from build123d import *

# Parameters (mm, degrees)
SKETCH1_R           = 3.048
BOSS_EXTRUDE1_DEPTH = 1.905
CUT_EXTRUDE1_DEPTH  = 1.651
BOSS_EXTRUDE2_START = 1.27
BOSS_EXTRUDE2_DEPTH = 1.27


with BuildPart() as part:
    # Sketch1 → Boss-Extrude1 (new body)
    with BuildSketch(Plane.XY):
        with BuildLine():
            Line((-5.49275, -17.49425), (-5.49275, -22.42185))
            Line((-5.49275, -22.42185), (-4.90855, -23.59025))
            Line((-4.90855, -23.59025), (-6.02615, -30.95625))
            ThreePointArc((-6.02615, -30.95625), (-5.598504604, -32.704973448), (-3.99415, -33.52165))
            ThreePointArc((-3.99415, -33.52165), (-0.284785682, -32.892281616), (3.42265, -32.25165))
            Line((3.42265, -32.25165), (4.94665, -24.09825))
            ThreePointArc((4.94665, -24.09825), (2.651841734, -25.057223226), (2.50825, -22.57425))
            ThreePointArc((2.50825, -22.57425), (2.10181036, -20.83747495), (2.73685, -19.17065))
            ThreePointArc((2.73685, -19.17065), (4.08470653, -17.176398636), (6.47065, -17.49425))
            ThreePointArc((6.47065, -17.49425), (7.46828342, -1.95088497), (5.45465, 13.49375))
            ThreePointArc((5.45465, 13.49375), (5.282315002, 20.474416107), (6.92785, 27.26055))
            ThreePointArc((6.92785, 27.26055), (5.106547792, 33.02758949), (-0.64135, 31.14675))
            Line((-0.64135, 31.14675), (-2.67335, 13.36675))
            Line((-2.67335, 13.36675), (-4.95935, 11.20775))
            Line((-4.95935, 11.20775), (-6.12775, -4.03225))
            Line((-6.12775, -4.03225), (-3.07975, -8.27405))
            Line((-3.07975, -8.27405), (-3.84175, -16.22425))
            Line((-3.84175, -16.22425), (-5.49275, -17.49425))
        make_face()
        with Locations(Location((3.16865, 29.24175, 0), (0, 0, 180))):
            Circle(SKETCH1_R, mode=Mode.SUBTRACT)
        with Locations(Location((-2.11455, -28.94965, 0), (0, 0, 180))):
            Circle(SKETCH1_R, mode=Mode.SUBTRACT)
    extrude(amount=BOSS_EXTRUDE1_DEPTH)

    # Sketch2 → Cut-Extrude1 (cut)
    with BuildSketch(Plane.XY.offset(1.905)):
        with BuildLine():
            Line((-7.059940767, -26.71445), (-7.49935, -23.51405))
            ThreePointArc((-7.49935, -23.51405), (-5.25575534, -22.137911475), (-3.94335, -19.85645))
            ThreePointArc((-3.94335, -19.85645), (-2.580214562, -13.534333063), (-2.16535, -7.08025))
            ThreePointArc((-2.16535, -7.08025), (-3.488996471, 2.074956789), (-4.95935, 11.20775))
            Line((-4.95935, 11.20775), (-2.67335, 13.36675))
            ThreePointArc((-2.67335, 13.36675), (-1.409957084, 3.210909205), (-0.455940767, -6.97865))
            ThreePointArc((-0.455940767, -6.97865), (-0.544530874, -12.566939921), (-1.471940767, -18.07845))
            ThreePointArc((-1.471940767, -18.07845), (-3.99586421, -22.571205419), (-7.059940767, -26.71445))
        make_face()
    extrude(amount=-CUT_EXTRUDE1_DEPTH, mode=Mode.SUBTRACT)

    # Sketch3 → Boss-Extrude2 (add)
    with BuildSketch(Plane.XY.offset(1.905).offset(BOSS_EXTRUDE2_START)):
        with BuildLine():
            Line((-5.49275, -17.49425), (-5.49275, -22.367063276))
            ThreePointArc((-5.49275, -22.367063276), (-4.541021091, -21.221008268), (-3.94335, -19.85645))
            ThreePointArc((-3.94335, -19.85645), (-2.580214562, -13.534333063), (-2.16535, -7.08025))
            ThreePointArc((-2.16535, -7.08025), (-3.488996471, 2.074956789), (-4.95935, 11.20775))
            Line((-4.95935, 11.20775), (-6.12775, -4.03225))
            Line((-6.12775, -4.03225), (-3.07975, -8.27405))
            Line((-3.07975, -8.27405), (-3.84175, -16.22425))
            Line((-3.84175, -16.22425), (-5.49275, -17.49425))
        make_face()
    extrude(amount=-BOSS_EXTRUDE2_DEPTH)


solid = part.part
Geometry: final body of the model. Coordinates: model frame, mm. A direction names the side the tool comes from. Round coordinates to 2 decimals unless told otherwise and drop trailing zeros. Loops run counter-clockwise (first coordinate to the right, second up) from the corner with the lowest first, then second, coordinate; pieces in that order, holes last. Notation, with made-up numbers: (13, 28) -> (22, 28) arc R30 ccw to (22, 57) -> close; hole circle Ø6 at (3.25, 3). An arc over 180 degrees is marked (long way). One line per question, with ' | ' between items. Start each with the question number.
1. Section A-A on z = 1.25. Count the separate pieces of the cut face and the enclosed holes in it, and give its area (3 significant figures).
2. Contact query for flat-ended pins moving along their axis: pin 1 (1.6 mm diameter, centred on y = -19.5, z = 1.5, fed in from -X); pin 2 (4 mm diameter, centred on x = 0, y = -8.5, fed in from +Z) (3 decimals); pin 3 (5 mm diameter, centred on x = 3.17, y = 29.24, fed in from +Z). Output: stop coordinate, or through.
3. Section D-D on y = -5.5. Output: boundary loops of the cut face in (x, z) (3 decimals).
4. Section B-B on y = -27. Output: boundary loops of the cut face in (x, z) (3 decimals), and give its area (3 significant figures).
5. Mould query, pull axis X, two halves, no side actions, for faces 4 (the face through (2.69, -25.08, 0.94)), 5 (the face through (2.1, -20.9, 0.9)), 6 (the face through (-3.455, -12.193, 1.61)). Classes: pulls with the +X half, pulls with the -X half, needs draft (parallel to the pull), parting line crosses it, or undercut.
6. Line query: line 1 along X through (y, z) = (-22, 0.9); line 2 along Z through (x, y) = (0.5, -1) (3 decimals); line 3 along X through (y, z) = (0, 1.5). Output: solid intervals per line, ascending. Write a range as [from, to].
7. Set-up query: faces 1 (the face through (-5.46, -27.22, 0.94)), 2 (the face through (7.475, -2.169, 0.939)), 3 (the face through (-3.074, -21.077, 1.091)). Return all of +Z, -Z, +X, -X, +Y, -Y with unobstructed straight access to the full face (end or side cutting, diameter ignored); none if empty.
8. Section C-C on x = 4. Output: boundary loops of the cut face in (y, z) (3 decimals).
Returned:
1) separate pieces: 2 | enclosed holes: 2 | area: 513 mm2
2) pin 1: stops at x = -5.49 | pin 2: stops at z = 1.905 | pin 3: passes through
3) outline: (-5.073, 0) -> (7.506, 0) -> (7.506, 1.905) -> (-0.575, 1.905) -> (-0.575, 0.254) -> (-2.383, 0.254) -> (-2.383, 3.175) -> (-5.073, 3.175) -> close
4) outline: (-5.426, 0) -> (-4.457, 0) -> (-4.457, 1.905) -> (-5.426, 1.905) -> close; (0.228, 0) -> (4.404, 0) -> (4.404, 1.905) -> (0.228, 1.905) -> close | area: 9.80 mm2
5) face 4: undercut | face 5: pulls with the +X half | face 6: pulls with the -X half
6) line 1: x = [-5.49, -5.13], [-3.63, 2.25] | line 2: z = [0, 1.905] | line 3: x = [-5.82, -3.18], [-1.08, 7.38]
7) face 1: +Z, -Z, -X | face 2: +Z, -Z, +X | face 3: +Z
8) outline: (-29.163, 0) -> (-25.19, 0) -> (-25.19, 1.905) -> (-29.163, 1.905) -> close; (-17.217, 0) -> (26.309, 0) -> (26.309, 1.905) -> (-17.217, 1.905) -> close; (32.174, 0) -> (33.414, 0) -> (33.414, 1.905) -> (32.174, 1.905) -> close
